Could you check a few things on this model? Use its own coordinates, in mm. Face numbers are marked on the shaded views. A direction names the side the tool comes from. Round coordinates to 2 decimals unless told otherwise and drop trailing zeros. Loops run counter-clockwise (first coordinate to the right, second up) from the corner with the lowest first, then second, coordinate; pieces in that order, holes last. Notation, with made-up numbers: (37, -38.75) - (86, -38.75) arc R11 ccw to (86, -21.75) - close; hole circle Ø4 at (83.25, 58). An arc over 180 degrees is marked (long way). Use one line per item in the form item = value.
```python
from build123d import *

# Parameters (mm, degrees)
SKETCH_1_W           = 150
SKETCH_1_H           = 123
SKETCH_1_R           = 1.5
EXTRUDE_1_DEPTH      = 3
SKETCH_2_W           = 150
SKETCH_2_H           = 6
EXTRUDE_2_DEPTH      = 17
SKETCH_3_W           = 75
SKETCH_3_H           = 6
EXTRUDE_3_DEPTH      = 37
SKETCH_4_W           = 150
SKETCH_4_H           = 111
EXTRUDE_4_DEPTH      = 3
SKETCH_6_W           = 10
SKETCH_6_H           = 123
CUT_EXTRUDE_1_DEPTH  = 50
SKETCH_7_W           = 3
SKETCH_7_H           = 101
EXTRUDE_5_DEPTH      = 17
SKETCH_9_W           = 75
SKETCH_9_H           = 6
EXTRUDE_6_DEPTH      = 37
CUT_EXTRUDE_2_DEPTH  = 37
SKETCH_12_R          = 5
CUT_EXTRUDE_3_DEPTH  = 3
CUT_EXTRUDE_5_DEPTH  = 6
SKETCH_14_R          = 5
CUT_EXTRUDE_6_DEPTH  = 3
SKETCH_15_W          = 140
SKETCH_15_H          = 3
CUT_EXTRUDE_7_DEPTH  = 6
SKETCH_17_W          = 140
SKETCH_17_H          = 6
SKETCH_17_W_2        = 3
SKETCH_17_H_2        = 101
EXTRUDE_7_DEPTH      = 17
SKETCH_19_W          = 140
SKETCH_19_H          = 1
CUT_EXTRUDE_10_DEPTH = 50
SKETCH_20_W          = 140
SKETCH_20_H          = 1
CUT_EXTRUDE_11_DEPTH = 50
SKETCH_21_W          = 3
SKETCH_21_H          = 101
CUT_EXTRUDE_12_DEPTH = 34
SKETCH_22_R          = 1.48
CUT_EXTRUDE_13_DEPTH = 10
EXTRUDE_START        = 1
SKETCH_23_R          = 5
SKETCH_23_R_2        = 2.6
EXTRUDE_8_DEPTH      = 1
SKETCH_24_R          = 5
SKETCH_24_R_2        = 2.6
EXTRUDE_9_DEPTH      = 1


with BuildPart() as part:
    # 草图1 → 凸台-拉伸1 (new body)
    with BuildSketch(Plane(origin=(0, 0, 0), x_dir=(1, 0, 0), z_dir=(0, 1, 0))):
        with Locations((75, 61.5)):
            Rectangle(SKETCH_1_W, SKETCH_1_H)
        with Locations(Location((19, 102.5, 0), (0, 0, 270))):
            Circle(SKETCH_1_R, mode=Mode.SUBTRACT)
        with Locations(Location((19, 20.5, 0), (0, 0, 270))):
            Circle(SKETCH_1_R, mode=Mode.SUBTRACT)
        with Locations(Location((141, 20.5, 0), (0, 0, 270))):
            Circle(SKETCH_1_R, mode=Mode.SUBTRACT)
        with Locations(Location((141, 102.5, 0), (0, 0, 270))):
            Circle(SKETCH_1_R, mode=Mode.SUBTRACT)
    extrude(amount=EXTRUDE_1_DEPTH)

    # 草图2 → 凸台-拉伸2 (add)
    with BuildSketch(Plane(origin=(0, 3, 0), x_dir=(1, 0, 0), z_dir=(0, 1, 0))):
        with Locations((75, 120)):
            Rectangle(SKETCH_2_W, SKETCH_2_H)
    extrude(amount=EXTRUDE_2_DEPTH)

    # 草图3 → 凸台-拉伸3 (add)
    with BuildSketch(Plane(origin=(0, 3, 0), x_dir=(1, 0, 0), z_dir=(0, 1, 0))):
        with Locations((112.5, 3)):
            Rectangle(SKETCH_3_W, SKETCH_3_H)
    extrude(amount=EXTRUDE_3_DEPTH)

    # 草图4 → 凸台-拉伸4 (add)
    with BuildSketch(Plane(origin=(0, 3, 0), x_dir=(1, 0, 0), z_dir=(0, 1, 0))):
        with Locations((75, 61.5)):
            Rectangle(SKETCH_4_W, SKETCH_4_H)
    extrude(amount=-EXTRUDE_4_DEPTH)

    # 草图6 → 切除-拉伸1 (cut)
    with BuildSketch(Plane.XZ):
        with Locations((145, -61.5)):
            Rectangle(SKETCH_6_W, SKETCH_6_H)
    extrude(amount=-CUT_EXTRUDE_1_DEPTH, mode=Mode.SUBTRACT)

    # 草图7 → 凸台-拉伸5 (add)
    with BuildSketch(Plane(origin=(0, 3, 0), x_dir=(1, 0, 0), z_dir=(0, 1, 0))):
        with Locations((1.5, 56.5)):
            Rectangle(SKETCH_7_W, SKETCH_7_H)
    extrude(amount=EXTRUDE_5_DEPTH)

    # 草图9 → 凸台-拉伸6 (add)
    with BuildSketch(Plane(origin=(0, 3, 0), x_dir=(1, 0, 0), z_dir=(0, 1, 0))):
        with Locations((37.5, 3)):
            Rectangle(SKETCH_9_W, SKETCH_9_H)
    extrude(amount=EXTRUDE_6_DEPTH)

    # 草图11 → 切除-拉伸2 (cut)
    with BuildSketch(Plane(origin=(0, 0, -6), x_dir=(-1, 0, 0), z_dir=(0, 0, -1))):
        with BuildLine():
            ThreePointArc((-107.6, 30), (-105, 27.4), (-102.4, 30))
            Line((-102.4, 30), (-107.6, 30))
        make_face()
        with BuildLine():
            Line((-107.6, 30), (-102.4, 30))
            ThreePointArc((-102.4, 30), (-105, 32.6), (-107.6, 30))
        make_face()
        with BuildLine():
            ThreePointArc((-32.4, 30), (-35, 32.6), (-37.6, 30))
            Line((-37.6, 30), (-32.4, 30))
        make_face()
        with BuildLine():
            Line((-32.4, 30), (-37.6, 30))
            ThreePointArc((-37.6, 30), (-35, 27.4), (-32.4, 30))
        make_face()
    extrude(amount=-CUT_EXTRUDE_2_DEPTH, mode=Mode.SUBTRACT)

    # 草图12 → 切除-拉伸3 (cut)
    with BuildSketch(Plane(origin=(0, 0, -6), x_dir=(-1, 0, 0), z_dir=(0, 0, -1))):
        with Locations((-105, 30)):
            Circle(SKETCH_12_R)
        with Locations((-35, 30)):
            Circle(SKETCH_12_R)
    extrude(amount=-CUT_EXTRUDE_3_DEPTH, mode=Mode.SUBTRACT)

    # 草图13 → 切除-拉伸5 (cut)
    with BuildSketch(Plane.XY.offset(-117)):
        with BuildLine():
            ThreePointArc((67.4, 10), (70, 7.4), (72.6, 10))
            Line((72.6, 10), (67.4, 10))
        make_face()
        with BuildLine():
            Line((67.4, 10), (72.6, 10))
            ThreePointArc((72.6, 10), (70, 12.6), (67.4, 10))
        make_face()
    extrude(amount=-CUT_EXTRUDE_5_DEPTH, mode=Mode.SUBTRACT)

    # 草图14 → 切除-拉伸6 (cut)
    with BuildSketch(Plane.XY.offset(-117)):
        with Locations((70, 10)):
            Circle(SKETCH_14_R)
    extrude(amount=-CUT_EXTRUDE_6_DEPTH, mode=Mode.SUBTRACT)

    # 草图15 → 切除-拉伸7 (cut)
    with BuildSketch(Plane.XY):
        with Locations((70, 38.5)):
            Rectangle(SKETCH_15_W, SKETCH_15_H)
    extrude(amount=-CUT_EXTRUDE_7_DEPTH, mode=Mode.SUBTRACT)

    # 草图17 → 凸台-拉伸7 (add)
    with BuildSketch(Plane(origin=(0, 20, 0), x_dir=(1, 0, 0), z_dir=(0, 1, 0))):
        with Locations((70, 120)):
            Rectangle(SKETCH_17_W, SKETCH_17_H)
        with Locations((1.5, 56.5)):
            Rectangle(SKETCH_17_W_2, SKETCH_17_H_2)
    extrude(amount=EXTRUDE_7_DEPTH)

    # 草图19 → 切除-拉伸10 (cut)
    with BuildSketch(Plane(origin=(0, 37, 0), x_dir=(1, 0, 0), z_dir=(0, 1, 0))):
        with Locations((70, 122.5)):
            Rectangle(SKETCH_19_W, SKETCH_19_H)
    extrude(amount=-CUT_EXTRUDE_10_DEPTH, mode=Mode.SUBTRACT)

    # 草图20 → 切除-拉伸11 (cut)
    with BuildSketch(Plane(origin=(0, 37, 0), x_dir=(1, 0, 0), z_dir=(0, 1, 0))):
        with Locations((70, 0.5)):
            Rectangle(SKETCH_20_W, SKETCH_20_H)
    extrude(amount=-CUT_EXTRUDE_11_DEPTH, mode=Mode.SUBTRACT)

    # 草图21 → 切除-拉伸12 (cut)
    with BuildSketch(Plane(origin=(0, 37, 0), x_dir=(1, 0, 0), z_dir=(0, 1, 0))):
        with Locations((1.5, 56.5)):
            Rectangle(SKETCH_21_W, SKETCH_21_H)
    extrude(amount=-CUT_EXTRUDE_12_DEPTH, mode=Mode.SUBTRACT)

    # 草图22 → 切除-拉伸13 (cut)
    with BuildSketch(Plane(origin=(0, 37, 0), x_dir=(1, 0, 0), z_dir=(0, 1, 0))):
        with Locations(Location((95, 119.5, 0), (0, 0, 270))):
            Circle(SKETCH_22_R)
        with Locations(Location((45, 119.5, 0), (0, 0, 270))):
            Circle(SKETCH_22_R)
        with Locations(Location((45, 3.5, 0), (0, 0, 270))):
            Circle(SKETCH_22_R)
        with Locations(Location((95, 3.5, 0), (0, 0, 270))):
            Circle(SKETCH_22_R)
    extrude(amount=-CUT_EXTRUDE_13_DEPTH, mode=Mode.SUBTRACT)

    # 草图23 → 凸台-拉伸8 (add)
    with BuildSketch(Plane.XY.offset(-120).offset(EXTRUDE_START)):
        with Locations((70, 10)):
            Circle(SKETCH_23_R)
        with Locations((70, 10)):
            Circle(SKETCH_23_R_2, mode=Mode.SUBTRACT)
    extrude(amount=-EXTRUDE_8_DEPTH)

    # 草图24 → 凸台-拉伸9 (add)
    # profile 1 of 2: a face of its own
    with BuildSketch(Plane(origin=(0, 0, -3), x_dir=(-1, 0, 0), z_dir=(0, 0, -1)).offset(EXTRUDE_START)):
        with Locations((-105, 30)):
            Circle(SKETCH_24_R)
        with Locations((-105, 30)):
            Circle(SKETCH_24_R_2, mode=Mode.SUBTRACT)
    # profile 2 of 2: a face of its own
    with BuildSketch(Plane(origin=(0, 0, -3), x_dir=(-1, 0, 0), z_dir=(0, 0, -1)).offset(EXTRUDE_START)):
        with Locations((-35, 30)):
            Circle(SKETCH_24_R)
        with Locations((-35, 30)):
            Circle(SKETCH_24_R_2, mode=Mode.SUBTRACT)
    extrude(amount=-EXTRUDE_9_DEPTH)


solid = part.part
```
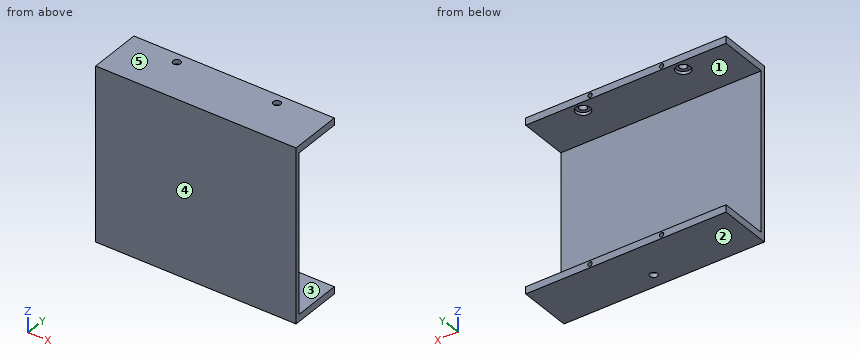
1. If we section it at B-B, the plane x = 105: Write out the boundary of the cut face in (y, z), plus the area to 3 significant figures.
Solution:
outline = (0, -122) - (37, -122) - (37, -117) - (3, -117) - (3, -6) - (25, -6) - (25, -4) - (27.4, -4) - (27.4, -1) - (0, -1) - close; (32.6, -4) - (35, -4) - (35, -6) - (37, -6) - (37, -1) - (32.6, -1) - close
area = 667 mm^2
2. We'd pull the mould along Z, two halves only. Please class the marked faces 3, 4 and 5: +Z half, -Z half, draft (parallel to the pull), parting line (faces both ways), or undercut.
Solution:
face_3 = undercut
face_4 = draft
face_5 = +Z half
3. On a 3-axis mill with a long thin cutter (end or side, diameter ignored), from which of +Z, -Z, +X, -X, +Y, -Y can I reach the whole of each face in a straight line? I mean the marked faces 1 and 2. Say none if no direction works.
Solution:
face_1 = +X, -X, +Y
face_2 = -Z, +X, -X, +Y, -Y
4. If we section it at C-C, the plane y = 18.5: Write out the boundary of the cut face in (x, z), plus the area to 3 significant figures.
Solution:
outline = (0, -122) - (140, -122) - (140, -117) - (0, -117) - close; (0, -6) - (140, -6) - (140, -1) - (0, -1) - close
area = 1,400 mm^2
5. For P1, Ø4, axis at x = 56, z = -91.5, coming from the +Y side; P2, Ø0.9, axis at x = 44.5, z = -3.5, coming from the +Y side, each with a flat end and sliding along its axis, tell me the tip position at first contact or that it passes through.
Solution:
P1 = 3
P2 = 27
6. Please list where these lines run through material, in increasing order: line 1 along Z through (x, y) = (95, 31); line 2 along Y through (x, z) = (105, -3.3); line 3 along Z through (x, y) = (82, 14).
Solution:
line_1 = -122 to -120.98, -118.02 to -117, -6 to -4.98, -2.02 to -1
line_2 = 0 to 27.4, 32.6 to 37
line_3 = -122 to -117, -6 to -1
7. If we section it at A-A, the plane y = 10: Write out the boundary of the cut face in (x, z).
Solution:
outline = (0, -122) - (67.4, -122) - (67.4, -119) - (65, -119) - (65, -117) - (0, -117) - close; (0, -6) - (140, -6) - (140, -1) - (0, -1) - close; (72.6, -122) - (140, -122) - (140, -117) - (75, -117) - (75, -119) - (72.6, -119) - close
